```python
from build123d import *

# Parameters (mm, degrees)
SKETCH1_R           = 1.65
SKETCH1_R_2         = 1.6
SKETCH1_R_3         = 2.2
SKETCH1_R_4         = 4
BOSS_EXTRUDE1_DEPTH = 7.5


with BuildPart() as part:
    # Sketch1 → Boss-Extrude1 (new body)
    with BuildSketch(Plane(origin=(0, 3.75, 0), x_dir=(1, 0, 0), z_dir=(0, 1, 0))):
        with BuildLine():
            Line((8, -68), (8, -15.81929202))
            ThreePointArc((8, -15.81929202), (7.249624617, -12.018707269), (5.111111111, -8.788495566))
            ThreePointArc((5.111111111, -8.788495566), (1.5, 0), (5.111111111, 8.788495566))
            ThreePointArc((5.111111111, 8.788495566), (7.249624617, 12.018707269), (8, 15.81929202))
            Line((8, 15.81929202), (8, 68))
            ThreePointArc((8, 68), (6.535533906, 71.535533906), (3, 73))
            Line((3, 73), (-22.5, 73))
            ThreePointArc((-22.5, 73), (-26.035533906, 71.535533906), (-27.5, 68))
            Line((-27.5, 68), (-27.5, -68))
            ThreePointArc((-27.5, -68), (-26.035533906, -71.535533906), (-22.5, -73))
            Line((-22.5, -73), (3, -73))
            ThreePointArc((3, -73), (6.535533906, -71.535533906), (8, -68))
        make_face()
        with Locations((0, -68)):
            Circle(SKETCH1_R, mode=Mode.SUBTRACT)
        with Locations((0, -52)):
            Circle(SKETCH1_R, mode=Mode.SUBTRACT)
        with Locations((0, 68)):
            Circle(SKETCH1_R, mode=Mode.SUBTRACT)
        with Locations((0, 52)):
            Circle(SKETCH1_R, mode=Mode.SUBTRACT)
        with Locations((-1.5, 15.5)):
            Circle(SKETCH1_R_2, mode=Mode.SUBTRACT)
        with Locations((-1.5, -15.5)):
            Circle(SKETCH1_R_2, mode=Mode.SUBTRACT)
        with Locations((-17.5, 0)):
            Circle(SKETCH1_R_3, mode=Mode.SUBTRACT)
        with Locations((0, -60)):
            Circle(SKETCH1_R_4, mode=Mode.SUBTRACT)
        with Locations((0, 60)):
            Circle(SKETCH1_R_4, mode=Mode.SUBTRACT)
        with Locations((-17.5, 60)):
            Circle(SKETCH1_R_3, mode=Mode.SUBTRACT)
        with Locations((-17.5, -60)):
            Circle(SKETCH1_R_3, mode=Mode.SUBTRACT)
    extrude(amount=-BOSS_EXTRUDE1_DEPTH)


solid = part.part
```
For this review, take the finished solid that the model builds, in its own axes (mm). A direction names the side the tool comes from. Round coordinates to 2 decimals unless told otherwise and drop trailing zeros. Write each loop counter-clockwise with the first axis right and the second up, starting at its lowest first coordinate (ties: lowest second). Pieces come first, ordered by that corner, then holes. Notation, with made-up numbers: (12, 67.5) - (45, 67.5) arc R25 ccw to (45, 87.5) - close; hole circle Ø2 at (16, -30.5). An arc over 180 degrees is marked (long way). Use CSV: the item, a comma, the result in double quotes.
1) Add section B-B on y = 2.5. Count the separate pieces of the cut face and the enclosed holes in it, and give its area (3 significant figures).
Conclusion:
separate pieces,"1"
enclosed holes,"11"
area,"4,860 mm^2"
2) Add section A-A on z = 52. Write out the cut boundary in (x, y), and give its area (4 significant figures).
Conclusion:
outline,"(-27.5, -3.75) - (-1.65, -3.75) - (-1.65, 3.75) - (-27.5, 3.75) - close; (1.65, -3.75) - (8, -3.75) - (8, 3.75) - (1.65, 3.75) - close"
area,"241.5 mm^2"
3) Add section C-C on z = 0. Write out the cut boundary in (x, y).
Conclusion:
outline,"(-27.5, -3.75) - (-19.7, -3.75) - (-19.7, 3.75) - (-27.5, 3.75) - close; (-15.3, -3.75) - (1.5, -3.75) - (1.5, 3.75) - (-15.3, 3.75) - close"
4) The part is to be moulded in two halves that separate along X. For faces 3 (the flat face through (-27.5, 0, -1)), 4 (the cylindrical face through (0.89, 0.05, -53.39)), 5 (the cylindrical face through (1.5, 0.1, 0.1)), 6 (the flat face through (-10, 0, -73)), say which applies: pulls with the +X half, pulls with the -X half, needs draft (parallel to the pull), parting line crosses it, or undercut.
Conclusion:
face 3,"pulls with the -X half"
face 4,"undercut"
face 5,"pulls with the +X half"
face 6,"needs draft"
5) Wall thickness on line 1 along Z through (x, y) = (-17.5, 1); line 2 along X through (y, z) = (-1.5, 68); line 3 along X through (y, z) = (1.5, 58): over which ranges is each line inside the solid? List them lowest first. Write a range as from..to.
Conclusion:
line 1,"z = -73..-62.2, -57.8..-2.2, 2.2..57.8, 62.2..73"
line 2,"x = -27.5..-1.65, 1.65..8"
line 3,"x = -27.5..-18.42, -16.58..-3.46, 3.46..8"
6) Clearance check with a flat-ended pin moving along its axis: pin 1 Ø3.5 at (x, z) = (-17.5, 0) entering from +Y. State where the tip first meets the part, or that it passes through.
Conclusion:
pin 1,"passes through"
7) For faces 1 (the cylindrical face through (-26.07, 0.05, 71.5)), 2 (the cylindrical face through (7.23, 0.05, -11.97)), list the 3-axis set-ups (+Z, -Z, +X, -X, +Y, -Y) from which the entire face can be reached by the end or side of a thin tool; tool diameter is ignored.
Conclusion:
face 1,"+Z, -X, +Y, -Y"
face 2,"+X, +Y, -Y"
